from build123d import *

# Parameters (mm, degrees)
BOSS_EXTRUDE1_DEPTH = 3
BOSS_EXTRUDE2_DEPTH = 30
CUT_EXTRUDE1_REACH  = 139.835
SKETCH3_R           = 1.8
CIRPATTERN1_COUNT   = 4


with BuildPart() as part:
    # Sketch1 → Boss-Extrude1 (new body)
    with BuildSketch(Plane(origin=(0, 0, 0), x_dir=(1, 0, 0), z_dir=(0, 1, 0))):
        Polygon((55.432771951, 22.961005942), (22.961005942, 55.432771951), (-22.961005942, 55.432771951), (-55.432771951, 22.961005942), (-55.432771951, -22.961005942), (-22.961005942, -55.432771951), (22.961005942, -55.432771951), (55.432771951, -22.961005942), align=None)
    extrude(amount=BOSS_EXTRUDE1_DEPTH)

    # Sketch2 → Boss-Extrude2 (add)
    with BuildSketch(Plane(origin=(0, 3, 0), x_dir=(1, 0, 0), z_dir=(0, 1, 0))):
        Polygon((55.432771951, -22.961005942), (55.432771951, 22.961005942), (22.961005942, 55.432771951), (-22.961005942, 55.432771951), (-55.432771951, 22.961005942), (-55.432771951, -22.961005942), (-22.961005942, -55.432771951), (22.961005942, -55.432771951), align=None)
        Polygon((52.432771951, -21.718365255), (52.432771951, 21.718365255), (21.718365255, 52.432771951), (-21.718365255, 52.432771951), (-52.432771951, 21.718365255), (-52.432771951, -21.718365255), (-21.718365255, -52.432771951), (21.718365255, -52.432771951), align=None, mode=Mode.SUBTRACT)
    extrude(amount=BOSS_EXTRUDE2_DEPTH)

    # Sketch3 → Cut-Extrude1 (cut, up to next)
    with BuildSketch(Plane(origin=(39.196888946, 0, 39.196888946), x_dir=(0.7071067811865475, 0, -0.7071067811865477), z_dir=(0.7071067811865477, 0, 0.7071067811865475)), mode=Mode.PRIVATE) as cut_extrude1_sk1:
        with Locations((-14, 16.5)):
            Circle(SKETCH3_R)
    cut_extrude1_tool1 = extrude(cut_extrude1_sk1.sketch, amount=-CUT_EXTRUDE1_REACH, mode=Mode.PRIVATE) & part.part
    # Sketch3 → Cut-Extrude1 (cut, up to next)
    with BuildSketch(Plane(origin=(39.196888946, 0, 39.196888946), x_dir=(0.7071067811865475, 0, -0.7071067811865477), z_dir=(0.7071067811865477, 0, 0.7071067811865475)), mode=Mode.PRIVATE) as cut_extrude1_sk2:
        with Locations((14, 16.5)):
            Circle(SKETCH3_R)
    cut_extrude1_tool2 = extrude(cut_extrude1_sk2.sketch, amount=-CUT_EXTRUDE1_REACH, mode=Mode.PRIVATE) & part.part
    cut_extrude1_1 = cut_extrude1_tool1.solids().sort_by_distance((29.297394, 16.5, 49.096384))[0]
    add(cut_extrude1_1, mode=Mode.SUBTRACT)
    cut_extrude1_2 = cut_extrude1_tool2.solids().sort_by_distance((49.096384, 16.5, 29.297394))[0]
    add(cut_extrude1_2, mode=Mode.SUBTRACT)
    cut_extrude1 = cut_extrude1_1 + cut_extrude1_2  # Cut-Extrude1 as one shape, for the pattern or mirror that repeats it

    # CirPattern1: Cut-Extrude1 ×4 about axis
    cirpattern1_axis = Axis((0, 0, 0), (0, 1, 0))
    for i in range(1, CIRPATTERN1_COUNT):
        add(cut_extrude1.rotate(cirpattern1_axis, i * 360 / CIRPATTERN1_COUNT), mode=Mode.SUBTRACT)


solid = part.part
Read the model definition and answer for the solid it produces. Units are mm, in the model's axes. A direction names the side the tool comes from. Coordinates: 2 decimals unless noted, no trailing zeros. Write each loop counter-clockwise with the first axis right and the second up, starting at its lowest first coordinate (ties: lowest second). Pieces come first, ordered by that corner, then holes. Notation, with made-up numbers: M 68,54.25 L 126,54.25 A25 ccw 126,72.25 Z; hole C -27.5,-7.5 d5. An arc over 180 degrees is marked long. Use a Markdown table: item, result.
Q1. Each of these flat-tipped pins is pushed along its axis until it touches: pin 1 Ø1.5 at (x, y) = (-42, 26.5) entering from +Z; pin 2 Ø1 at (y, z) = (15.5, 41.5) entering from -X. Where does it stop, or does it pass through?
Answer block:
| item | result |
|---|---|
| pin 1 | stops at z = 37.14 |
| pin 2 | stops at x = -37.39 |
Q2. Determine the mould class of faces 1 (the face through (-47.366, 18.018, 28.936)), 2 (the face through (55.433, 16, 0)), 3 (the face through (-1, 0, -1)) for opening direction X: released by +X, released by -X, zero draft, split by the parting line, or undercut.
Answer block:
| item | result |
|---|---|
| face 1 | undercut |
| face 2 | released by +X |
| face 3 | zero draft |
Q3. The part is cut by section A-A, the plane y = 12.5. Write down the section's boundary in (x, z), then the cut area to 3 significant figures.
Answer block:
| item | result |
|---|---|
| outline | M -55.43,-22.96 L -22.96,-55.43 L 22.96,-55.43 L 55.43,-22.96 L 55.43,22.96 L 22.96,55.43 L -22.96,55.43 L -55.43,22.96 Z; hole M -52.43,-21.72 L -21.72,-52.43 L 21.72,-52.43 L 52.43,-21.72 L 52.43,21.72 L 21.72,52.43 L -21.72,52.43 L -52.43,21.72 Z |
| area | 1,070 mm2 |
Q4. Which of the six approach directions +Z, -Z, +X, -X, +Y, -Y give full straight-line access (tool end or side, diameter ignored) to faces 4 (the face through (-36.86, 17.79, -37.29)), 5 (the face through (0, 16, 55.433))?
Answer block:
| item | result |
|---|---|
| face 4 | +Y |
| face 5 | +Z, +X, -X, +Y, -Y |
Q5. The part is cut by section B-B, the plane z = 17. Write down the section's boundary in (x, y), then the cut area to 3 significant figures.
Answer block:
| item | result |
|---|---|
| outline | M -55.43,0 L 55.43,0 L 55.43,33 L 52.43,33 L 52.43,3 L -52.43,3 L -52.43,33 L -55.43,33 Z |
| area | 513 mm2 |
Q6. Straight lines are drawn through the part: L1, parallel to Z at x = 0, y = 14; L2, parallel to Z at x = 24, y = 4. For each, find the intervals that lie inside material, in ascending order. Write a range as [from, to].
Answer block:
| item | result |
|---|---|
| L1 | z = [-55.43, -52.43], [52.43, 55.43] |
| L2 | z = [-54.39, -50.15], [50.15, 54.39] |
Q7. The part is cut by section C-C, the plane x = -10.5. Write down the section's boundary in (y, z), then the cut area to 3 significant figures.
Answer block:
| item | result |
|---|---|
| outline | M 0,-55.43 L 33,-55.43 L 33,-52.43 L 3,-52.43 L 3,52.43 L 33,52.43 L 33,55.43 L 0,55.43 Z |
| area | 513 mm2 |
